The drawing under review shows one solid part. Ordinate dimensions are in mm from its lowest x, y, z. A direction names the side the tool comes from. Give positions to 0.01 mm unless a question says otherwise; leave off trailing zeros. Loops run counter-clockwise (first coordinate to the right, second up) from the corner with the lowest first, then second, coordinate; pieces in that order, holes last. Notation, with made-up numbers: (-5.5, 23.25) - (42.5, 23.25) arc R19 cw to (42.5, 46.25) - close; hole circle Ø8 at (86.5, -13). An arc over 180 degrees is marked (long way). One line per item, written item: value. Start each with the question number.
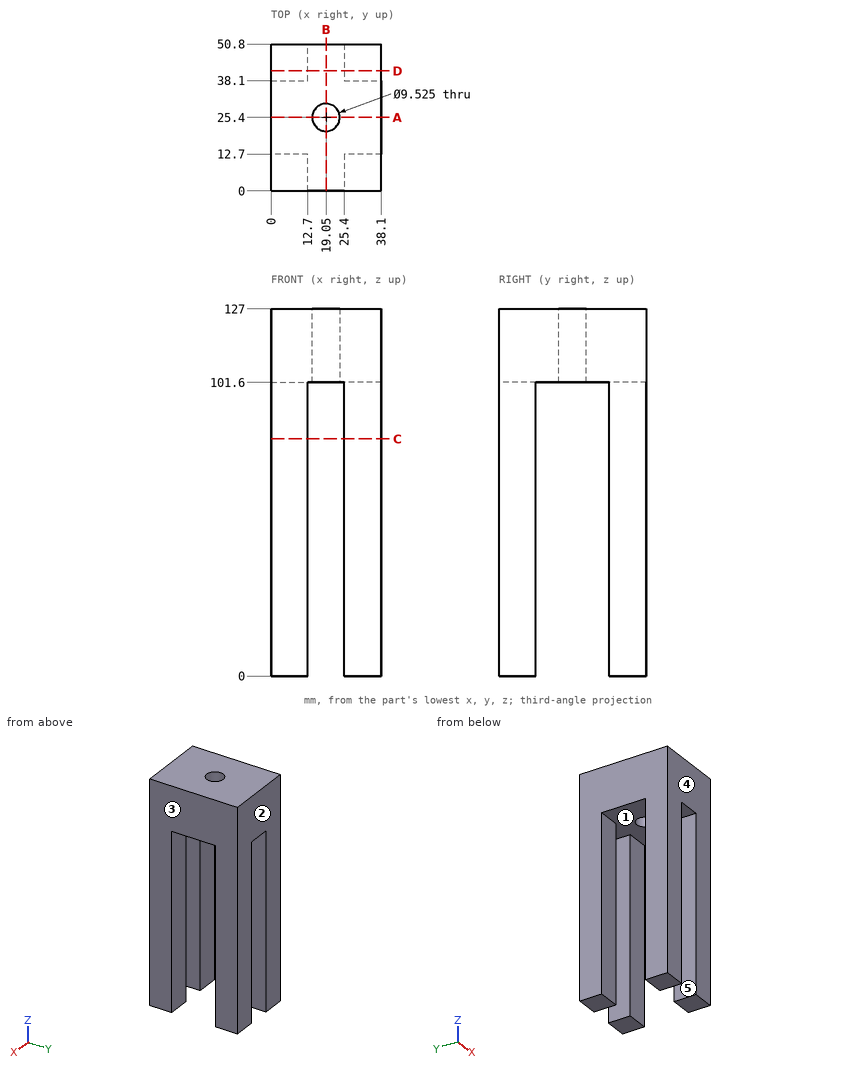
(1) Machinability: for the marked faces 4 and 5, which of the approach directions +Z, -Z, +X, -X, +Y, -Y give a long, thin tool a straight path to every point of the face, cutting with its end or side? Answer none if there is none.
(2) Take a section at D-D on y = 41.5. State the section outline as (x, z) points, and give its area (3 significant figures).
(3) Draft analysis for pull direction X (two halves, no side actions). For the marked faces 1, 2 and 3, state which applies: pulls with the +X half, pulls with the -X half, needs draft (parallel to the pull), parting line crosses it, or undercut.
(4) Take a section at B-B on x = 19.05. State the section outline as (y, z) points.
(5) Take a section at C-C on z = 82. State the section outline as (x, y) points, and give its area (3 significant figures).
(6) For pin 1 Ø1.5 at (y, z) = (27.5, 101) entering from +X; pin 2 Ø10 at (x, z) = (18.5, 40.5) entering from +Y, all flat-tipped, find the tip position at first contact; note any pin that passes through.
(7) To check wall thickness, follow L1, parallel to X at y = 5, z = 39; L2, parallel to X at y = 25, z = 110; L3, parallel to Y at x = 19.05, z = 113.5. State the ranges of each line that lie inside material, in increasing order. Write a range as from..to.
(8) Take a section at A-A on y = 25.4. State the section outline as (x, z) points, and give its area (3 significant figures).
Here are the results:
1. face 4: +Z, -Z, +X, -X, -Y
1. face 5: -Z, +Y, -Y
2. outline: (0, 0) - (12.7, 0) - (12.7, 101.6) - (25.4, 101.6) - (25.4, 0) - (38.1, 0) - (38.1, 127) - (0, 127) - close
2. area: 3,550 mm²
3. face 1: undercut
3. face 2: needs draft
3. face 3: pulls with the +X half
4. outline: (0, 101.6) - (20.64, 101.6) - (20.64, 127) - (0, 127) - close; (30.16, 101.6) - (50.8, 101.6) - (50.8, 127) - (30.16, 127) - close
5. outline: (0, 0) - (12.7, 0) - (12.7, 12.7) - (0, 12.7) - close; (0, 38.1) - (12.7, 38.1) - (12.7, 50.8) - (0, 50.8) - close; (25.4, 0) - (38.1, 0) - (38.1, 12.7) - (25.4, 12.7) - close; (25.4, 38.1) - (38.1, 38.1) - (38.1, 50.8) - (25.4, 50.8) - close
5. area: 645 mm²
6. pin 1: x = 38.1
6. pin 2: through
7. L1: 0..12.7, 25.4..38.1
7. L2: 0..14.3, 23.8..38.1
7. L3: 0..20.64, 30.16..50.8
8. outline: (0, 101.6) - (14.29, 101.6) - (14.29, 127) - (0, 127) - close; (23.81, 101.6) - (38.1, 101.6) - (38.1, 127) - (23.81, 127) - close
8. area: 726 mm²
